The listing builds one solid part. Answer for the finished solid, in the listing's coordinates (mm). Give positions to 0.01 mm unless a question says otherwise; leave off trailing zeros. Order: outer loops, then holes, each group sorted by start corner. A loop starts at its lowest first (then second) coordinate and runs counter-clockwise, first axis right, second up. Notation, with made-up numbers: (16.25, -33.75) - (27.25, -33.75) arc R22 cw to (27.25, -19.75) - close; hole circle Ø4 at (30.5, 64.25). An arc over 180 degrees is marked (long way). Answer in a Markdown table with one row per item. Add a question column.
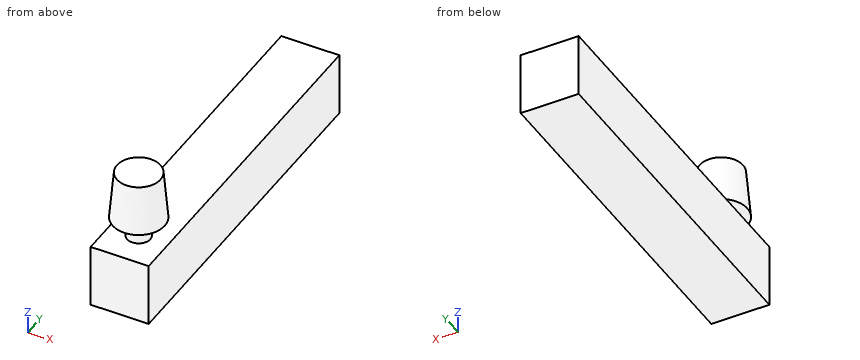
Autodesk Inventor part; units mm, degrees
ref_plane "YZ Plane" through (0, 0, 0) normal (1, 0, 0) x (0, 1, 0)
ref_plane "XZ Plane" through (0, 0, 0) normal (0, 1, 0) x (-1, 0, 0)
ref_plane "XY Plane" through (0, 0, 0) normal (0, 0, 1) x (1, 0, 0)
sketch "Sketch1" plane through (0, 0, 0) normal (0, 0, 1) x (1, 0, 0)
  line L0 (0, 0) -> (20, 0)
  line L1 (20, 0) -> (20, 120)
  line L2 (20, 120) -> (0, 120)
  line L3 (0, 120) -> (0, 0)
  dimension "d0" = 120
  dimension "d1" = 20
extrude "Extrusion1" add sketch "Sketch1" along normal blind 22
sketch "Sketch2" plane through (0, 0, 22) normal (0, 0, 1) x (1, 0, 0)
  point P0 (0, 0)
sketch "Sketch3" plane through (0, 0, 22) normal (0, 0, 1) x (1, 0, 0)
  circle A0 centre (10, 12) radius 4
  line L0 (0, 0) -> (20, 0) construction
  line L1 (10, 12) -> (10, 0) construction
  dimension "d4" = 12
  dimension "d5" = 8
extrude "Extrusion2" add sketch "Sketch3" along normal blind 7
sketch "Sketch4" plane through (10, 12, 29) normal (0, 0, 1) x (1, 0, 0)
  circle A0 centre (0, 0) radius 4 construction
  circle A1 centre (0, 0) radius 9
  point P0 (-10, -12)
  dimension "d8" = 18
extrude "Extrusion3" add sketch "Sketch4" along normal blind 17 draft -5
properties part number "FlowMeter"
(1) Each of these flat-tipped pins is pushed along its axis until it touches: P1, Ø6, axis at x = 9, y = 71.5, coming from the +Z side; P2, Ø6, axis at x = 13, y = 100, coming from the -Z side; P3, Ø12, axis at x = 5, z = 35, coming from the +Y side. Where does it stop, or does it pass through?
(2) Find section B-B, the plane x = 10. Write down the section's boundary in (y, z), plus the area to 3 significant figures.
(3) Straight lines are drawn through the part: line 1 (Z direction, x = 15.25, y = 9.5); line 2 (Z direction, x = 14, y = 51.5); line 3 (Y direction, x = 10.25, z = 32). For each, find the intervals that lie inside material, in ascending order.
(4) Find section C-C, the plane y = 50.5. Write down the section's boundary in (x, z), plus the area to 3 significant figures.
(5) Find section A-A, the plane y = 12. Write down the section's boundary in (x, z).
Answer key:
| question | item | result |
|---|---|---|
| 1 | P1 | z = 22 |
| 1 | P2 | z = 0 |
| 1 | P3 | y = 20.81 |
| 2 | outline | (0, 0) - (120, 0) - (120, 22) - (16, 22) - (16, 29) - (21, 29) - (19.51, 46) - (4.49, 46) - (3, 29) - (8, 29) - (8, 22) - (0, 22) - close |
| 2 | area | 2,980 mm² |
| 3 | line 1 | 0 to 22, 29 to 46 |
| 3 | line 2 | 0 to 22 |
| 3 | line 3 | 3.27 to 20.73 |
| 4 | outline | (0, 0) - (20, 0) - (20, 22) - (0, 22) - close |
| 4 | area | 440 mm² |
| 5 | outline | (0, 0) - (20, 0) - (20, 22) - (14, 22) - (14, 29) - (19, 29) - (17.51, 46) - (2.49, 46) - (1, 29) - (6, 29) - (6, 22) - (0, 22) - close |
